Geometry: final body of the model. Coordinates: model frame, mm. A direction names the side the tool comes from. Give positions to 0.01 mm unless a question says otherwise; leave off trailing zeros. Write each loop counter-clockwise with the first axis right and the second up, starting at its lowest first coordinate (ties: lowest second). Pieces come first, ordered by that corner, then holes.
Q1. Line query: L1, parallel to Z at x = -5.5, y = 3; L2, parallel to X at y = 11, z = -7; L3, parallel to X at y = -1, z = 12.75. Output: solid intervals per line, ascending.
Q2. Cut plane B-B on x = -5.5. Return the cut outline in (y, z).
Q3. Cut plane D-D on z = -12.25. Return the cut outline in (x, y).
Q4. Cut plane C-C on y = 12.5. Return the cut outline in (x, z), plus the area to 3 significant figures.
Q5. Reachability of faces 1 (the face through (5.27, -9.66, 2.18)), 2 (the face through (7.19, -13.17, 0.21)) from +Z, -Z, +X, -X, +Y, -Y: full face, straight path, thin tool, end or side. Return the list, or none.
Q6. Draft query along X for faces 3 (the face through (-15, 0, 0)), 4 (the face through (6, 10, 15)), 5 (the face through (2, 0, -11)). Return one class per face: pulls with the +X half, pulls with the -X half, needs draft (parallel to the pull), parting line crosses it, or undercut.
Q7. Pin query (flat end, axial travel): pin 1 (1.5 mm diameter, centred on y = 16.5, z = -1.5, fed in from +X); pin 2 (2 mm diameter, centred on x = 20, z = -11.5, fed in from +Y); pin 3 (13 mm diameter, centred on y = 7, z = -2.5, fed in from +X). Return the tip coordinate at first contact, or that it passes through.
Q8. Cut plane A-A on z = 4.5. Return the cut outline in (x, y), plus the area to 3 significant figures.
```python
from build123d import *

# Parameters (mm, degrees)
EXTRUDE_1_DEPTH = 15
SHELL_1_T       = -4


with BuildPart() as part:
    # 草图1 → 凸台-拉伸1 (new, symmetric)
    with BuildSketch(Plane.XY):
        Polygon((30, 0), (-15, 25.980762114), (-15, -25.980762114), align=None)
    extrude(amount=EXTRUDE_1_DEPTH, both=True)

    # 抽壳1
    shell_1_openings = [part.faces().sort_by_distance(p)[0] for p in [
        (0, 0, 15),
    ]]
    offset(amount=SHELL_1_T, openings=shell_1_openings, kind=Kind.INTERSECTION)


solid = part.part
```
Data:
1. L1: z = -15 to -11
1. L2: x = -15 to -11, 2.95 to 10.95
1. L3: x = -15 to -11, 20.27 to 28.27
2. outline: (-20.5, -15) - (20.5, -15) - (20.5, 15) - (15.88, 15) - (15.88, -11) - (-15.88, -11) - (-15.88, 15) - (-20.5, 15) - close
3. outline: (-15, -25.98) - (30, 0) - (-15, 25.98) - close
4. outline: (-15, -15) - (8.35, -15) - (8.35, 15) - (0.35, 15) - (0.35, -11) - (-11, -11) - (-11, 15) - (-15, 15) - close
4. area: 405 mm2
5. face 1: +Z
5. face 2: +Z, -Z, +X, -Y
6. face 3: pulls with the -X half
6. face 4: needs draft
6. face 5: undercut
7. pin 1: stops at x = 2.72
7. pin 2: stops at y = 6.35
7. pin 3: stops at x = 29.13
8. outline: (-15, -25.98) - (30, 0) - (-15, 25.98) - close; hole (-11, -19.05) - (22, 0) - (-11, 19.05) - close
8. area: 540 mm2
